Build history of the part. All positions in model axes, mm. A direction names the side the tool comes from. Round coordinates to 2 decimals unless told otherwise and drop trailing zeros. Loops run counter-clockwise (first coordinate to the right, second up) from the corner with the lowest first, then second, coordinate; pieces in that order, holes last. Notation, with made-up numbers: (73.5, 54) -> (98.5, 54) arc R32 cw to (98.5, 83) -> close; hole circle Ø7 at (-14.5, 83). An arc over 180 degrees is marked (long way). Put each result on its own line as item: value. Start each with the question number.
Autodesk Inventor part; units mm, degrees
ref_plane "YZ Plane" through (0, 0, 0) normal (1, 0, 0) x (0, 1, 0)
ref_plane "XZ Plane" through (0, 0, 0) normal (0, 1, 0) x (-1, 0, 0)
ref_plane "XY Plane" through (0, 0, 0) normal (0, 0, 1) x (1, 0, 0)
sketch "Sketch1" plane through (0, 0, 0) normal (0, 0, 1) x (1, 0, 0)
  line L0 (0, 0) -> (0, 70)
  line L1 (0, 70) -> (15, 70)
  line L2 (15, 70) -> (15, 45)
  line L3 (15, 45) -> (95, 45)
  line L4 (95, 45) -> (95, 55)
  line L5 (95, 55) -> (100, 55)
  line L6 (100, 55) -> (100, 40)
  line L7 (100, 40) -> (15, 0)
  line L8 (15, 0) -> (0, 0)
  line L9 (100, 40) -> (95, 45) construction
  line L10 (15, 35) -> (65.8896, 35)
  line L11 (65.8896, 35) -> (15, 11.0519)
  line L12 (15, 11.0519) -> (15, 35)
  dimension "d0" = 5
  dimension "d1" = 80
  dimension "d2" = 70
  dimension "d3" = 25
  dimension "d4" = 15
  dimension "d5" = 15
  dimension "d6" = 10
  dimension "d7" = 135
  dimension "d8" = 10
  dimension "d9" = 10
  dimension "d10" = 15
extrude "Extrusion1" add sketch "Sketch1" along normal blind 20
sketch "Sketch2" plane through (15, 11.0519, 0) normal (1, 0, 0) x (0, 0, -1)
  line L0 (0, 0) -> (0, 23.9481)
  line L1 (0, 23.9481) -> (-20, 23.9481)
  line L2 (-20, 0) -> (-20, 23.9481)
  line L3 (0, 0) -> (-20, 0)
  circle A0 centre (-10, 11.974) radius 4
  line L4 (0, 23.9481) -> (-20, 23.9481) construction
  line L5 (-10, 23.9481) -> (-10, 0) construction
  point P0 (0, -11.0519)
  dimension "d14" = 8
extrude "Extrusion2" cut sketch "Sketch2" along normal blind 71.75 contours A0
hole "Hole1" at (15, 23.026, 10) direction (-1, 0, 0) diameter 3.4036 end through all counterbore diameter 6.5024 counterbore depth 3.4036
sketch "Sketch3" plane through (15, 45, 0) normal (1, 0, 0) x (0, 0, -1)
  line L0 (0, 0) -> (0, 25)
  line L1 (0, 25) -> (-20, 25)
  line L2 (-20, 0) -> (-20, 25)
  line L3 (0, 0) -> (-20, 0)
  circle A0 centre (-10, -36.7642) radius 38.1
  point P0 (0, -45)
  dimension "d28" = 76.2
extrude "Extrusion3" add sketch "Sketch3" along normal up to surface (80 mm away) contours L3 A0 picked at (-11.1228, 0.3955)
fillet "Fillet1" radius 2.5 7 edges at (15, 70, 10) (0, 70, 10) (95, 55, 10) (100, 55, 10) (0, 0, 10) (15, 0, 10) (100, 40, 10)
equation "\"d4\" = d5"
equation "\"d10\" = d5"
equation "\"d14\" = d13"
properties part number "Spool Holder"
Item 1: Cut at C-C on x = 30. Write the cut outline in (y, z), then the cut area to 3 significant figures.
Item 2: Cut at A-A on x = 49. Write the cut outline in (y, z).
Item 3: Pull direction Z, two halves, no side cores. Call faces 5 (the face through (54.44, 46.336, 10.142)), 6 (the face through (15, 20, 8)), 7 (the face through (13.3, 26.2, 10.7)): +Z half, -Z half, draft (parallel to the pull), parting line (faces both ways), or undercut.
Item 4: Drop flat-ended pins along their axis: pin 1 (10 mm diameter, centred on x = 39, z = 6, fed in from +Y); pin 2 (2 mm diameter, centred on x = 70.5, z = 10.5, fed in from -Y); pin 3 (6 mm diameter, centred on x = 45.5, z = 12, fed in from -Y). Give the stop position or say it passes through.
Item 5: Wall check: line 1 (X direction, y = 49, z = 5); line 2 (Y direction, x = 12.8, z = 10); line 3 (X direction, y = 58.5, z = 6). Give the ranges that are in metal, low to high. Write a range as from..to.
Item 6: 3-axis set-ups, long thin cutter, end or side, ignore diameter. For faces 1 (the face through (40, 35, 10)), 2 (the face through (11.596, 24.4, 8.6)), 3 (the face through (95.752, 54.287, 10.14)), 4 (the face through (5.717, 24.687, 10.369)): which of +Z, -Z, +X, -X, +Y, -Y reach the whole face in a straight line?
Ans:
1. outline: (7.06, 0) -> (18.11, 0) -> (18.11, 20) -> (7.06, 20) -> close; (35, 0) -> (45, 0) arc R38.1 ccw to (45, 20) -> (35, 20) -> close
1. area: 439 mm2
2. outline: (16, 0) -> (27.05, 0) -> (27.05, 20) -> (16, 20) -> close; (35, 0) -> (45, 0) arc R38.1 ccw to (45, 20) -> (35, 20) -> close; hole circle Ø8 at (23.03, 10)
3. face 5: parting line
3. face 6: draft
3. face 7: undercut
4. pin 1: stops at y = 46.34
4. pin 2: stops at y = 26.73
4. pin 3: stops at y = 12.94
5. line 1: x = 0..15, 95..100
5. line 2: y = 0..19.77, 26.28..69.98
5. line 3: x = 0..15
6. face 1: +Z, -Z
6. face 2: +X
6. face 3: +Z, -Z, +Y
6. face 4: +X, -X
